```python
from build123d import *

# Parameters (mm, degrees)
SKETCH1_W           = 87.47
SKETCH1_H           = 9.7
BOSS_EXTRUDE1_DEPTH = 3.175
SKETCH3_R           = 1.415
CUT_EXTRUDE1_DEPTH  = 10
CUT_EXTRUDE2_DEPTH  = 10


with BuildPart() as part:
    # Sketch1 → Boss-Extrude1 (new body)
    with BuildSketch(Plane.XY):
        Rectangle(SKETCH1_W, SKETCH1_H)
    extrude(amount=BOSS_EXTRUDE1_DEPTH)

    # Sketch3 → Cut-Extrude1 (cut)
    with BuildSketch(Plane.XY.offset(3.175)):
        with Locations((-40.553019485, 1.668019485)):
            Circle(SKETCH3_R)
        with Locations((0, 1.668019485)):
            Circle(SKETCH3_R)
        with Locations((40.553019485, 1.668019485)):
            Circle(SKETCH3_R)
    extrude(amount=-CUT_EXTRUDE1_DEPTH, mode=Mode.SUBTRACT)

    # Sketch4 → Cut-Extrude2 (cut)
    with BuildSketch(Plane.XY.offset(3.175)):
        Polygon((0, -1.93), (-43.735, -1.93), (-43.735, -4.85), (43.735, -4.85), (43.735, -1.93), align=None)
    extrude(amount=-CUT_EXTRUDE2_DEPTH, mode=Mode.SUBTRACT)


solid = part.part
```
Part model, mm, in its own coordinate system. Round coordinates to 2 decimals unless told otherwise and drop trailing zeros. Order: outer loops, then holes, each group sorted by start corner. A loop starts at its lowest first (then second) coordinate and runs counter-clockwise, first axis right, second up. Notation, with made-up numbers: M 14.25,-10.75 L 41.25,-10.75 A26 ccw 41.25,7.25 Z; hole C 89.25,7 d11. An arc over 180 degrees is marked long. Answer in a Markdown table with one row per item. Add a question column.
Q1. Mould opens along Y. For faces 1 (the face through (-1, 3, 0)), 2 (the face through (-1, 4.85, 2)), 3 (the face through (-39.246, 1.126, 1.61)) say: +Y half, -Y half, draft (parallel to the pull), parting line (faces both ways), or undercut.
Q2. Wall check: L1, parallel to X at y = 1.75, z = 2.4 (3 decimals); L2, parallel to Y at x = 0, z = 2.15; L3, parallel to X at y = 0.75, z = 1.05 (3 decimals). Give the ranges that are in metal, low to high. Write a range as from..to.
Q3. Pin check, flat tip, straight feed: pin 1 (1.7 mm diameter, centred on x = 0, y = 1.67, fed in from -Z). Stop position of the tip, or through.
Q4. Cut at A-A on x = 0. Give the cut face in (y, z) (3 decimals), and give its area (3 significant figures).
Q5. Cut at B-B on z = 2.6. Give the cut face in (x, y) (3 decimals), and give its area (3 significant figures).
Established:
| question | item | result |
|---|---|---|
| 1 | face 1 | draft |
| 1 | face 2 | +Y half |
| 1 | face 3 | undercut |
| 2 | L1 | x = -43.735..-41.966, -39.14..-1.413, 1.413..39.14, 41.966..43.735 |
| 2 | L2 | y = -1.93..0.25, 3.08..4.85 |
| 2 | L3 | x = -43.735..-41.63, -39.476..-1.077, 1.077..39.476, 41.63..43.735 |
| 3 | pin 1 | passes through |
| 4 | outline | M -1.93,0 L 0.253,0 L 0.253,3.175 L -1.93,3.175 Z; M 3.083,0 L 4.85,0 L 4.85,3.175 L 3.083,3.175 Z |
| 4 | area | 12.5 mm2 |
| 5 | outline | M -43.735,-1.93 L 43.735,-1.93 L 43.735,4.85 L -43.735,4.85 Z; hole C -40.553,1.668 d2.83; hole C 0,1.668 d2.83; hole C 40.553,1.668 d2.83 |
| 5 | area | 574 mm2 |
